```python
from build123d import *

# Parameters (mm, degrees)
BASPROSKE_W         = 2
BASPROSKE_H         = 32
TOOTHCUT_DEPTH      = 46.299006612
TEETHCUTS_COUNT     = 30
TEETHCUTS_ANGLE     = 348
BORSKE_R            = 0.4
BORE_DEPTH          = 50.0000508
CUT_EXTRUDE_1_DEPTH = 10
CUT_EXTRUDE_3_DEPTH = 46.215730311
EXTRUDE_1_DEPTH     = 2
SKETCH_5_R          = 2
CUT_EXTRUDE_4_DEPTH = 10
EXTRUDE_START       = -2
EXTRUDE_2_DEPTH     = 2
SKETCH_8_R          = 2
CUT_EXTRUDE_6_DEPTH = 2
SKETCH_9_R          = 1.5
EXTRUDE_3_DEPTH     = 2
FILLET_7_R          = 2
CUT_EXTRUDE_7_DEPTH = 10
FILLET_8_R          = 2
FILLET_9_R          = 1


with BuildPart() as part:
    # BasProSke → Base-Revolve (revolve)
    with BuildSketch(Plane(origin=(0, 0, 0), x_dir=(1, 0, 0), z_dir=(0, 1, 0)), mode=Mode.PRIVATE) as base_revolve_sk:
        with Locations((1, 16)):
            Rectangle(BASPROSKE_W, BASPROSKE_H)
    revolve(base_revolve_sk.sketch.rotate(Axis((-10, 0, 0), (1, 0, 0)), 180), axis=Axis((-10, 0, 0), (1, 0, 0)))

    # TooCutSke → ToothCut (cut, through all)
    with BuildSketch(Plane(origin=(0, 0, 0), x_dir=(0, 0, -1), z_dir=(1, 0, 0))):
        with BuildLine():
            ThreePointArc((0.918551563, 27.483654488), (0, 27.499), (-0.918551563, 27.483654488))
            ThreePointArc((-0.918551563, 27.483654488), (-1.617208176, 29.787801627), (-2.761784709, 31.906093311))
            ThreePointArc((-2.761784709, 31.906093311), (0, 32.0254), (2.761784709, 31.906093311))
            ThreePointArc((2.761784709, 31.906093311), (1.617208176, 29.787801627), (0.918551563, 27.483654488))
        make_face()
    toothcut = extrude(amount=TOOTHCUT_DEPTH, mode=Mode.SUBTRACT)

    # TeethCuts: ToothCut ×30 about axis
    teethcuts_axis = Axis((-10, 0, 0), (1, 0, 0))
    for i in range(1, TEETHCUTS_COUNT):
        add(toothcut.rotate(teethcuts_axis, i * TEETHCUTS_ANGLE / (TEETHCUTS_COUNT - 1)), mode=Mode.SUBTRACT)

    # BorSke → Bore (cut, symmetric)
    with BuildSketch(Plane(origin=(0, 0, 0), x_dir=(0, 0, -1), z_dir=(1, 0, 0))):
        with Locations(Location((0, 0, 0), (0, 0, 180))):
            Circle(BORSKE_R)
    extrude(amount=BORE_DEPTH, both=True, mode=Mode.SUBTRACT)

    # 草图1 → 切除-拉伸1 (cut)
    with BuildSketch(Plane(origin=(2, 0, 0), x_dir=(0, 0, -1), z_dir=(1, 0, 0))):
        Polygon((3.344910825, 31.824700652), (-3.960111671, -37.677945718), (64.810502564, -34.553326749), (47.008100667, 53.868547869), (5.993727235, 38.229973826), align=None)
    extrude(amount=-CUT_EXTRUDE_1_DEPTH, mode=Mode.SUBTRACT)

    # 草图2 → 切除-拉伸3 (cut, through all)
    with BuildSketch(Plane(origin=(2, 0, 0), x_dir=(0, 0, -1), z_dir=(1, 0, 0))):
        with BuildLine():
            Line((4.939512658, 27.051732213), (6.979218814, 36.725980442))
            Line((6.979218814, 36.725980442), (-6.447162529, 36.725980442))
            Line((-6.447162529, 36.725980442), (-5.501449664, 26.943070586))
            ThreePointArc((-5.501449664, 26.943070586), (-0.286173264, 27.497510903), (4.939512658, 27.051732213))
        make_face()
        with BuildLine():
            Line((-11.106203944, -25.156455135), (-12.164876938, -35.534369935))
            Line((-12.164876938, -35.534369935), (-0.063712698, -31.064954068))
            Line((-0.063712698, -31.064954068), (0, -27.499))
            ThreePointArc((0, -27.499), (-5.675281546, -26.906991292), (-11.106203944, -25.156455135))
        make_face()
    extrude(amount=-CUT_EXTRUDE_3_DEPTH, mode=Mode.SUBTRACT)

    # 草图4 → 凸台-拉伸1 (add)
    with BuildSketch(Plane(origin=(2, 0, 0), x_dir=(0, 0, -1), z_dir=(1, 0, 0))):
        Polygon((2.874428211, 27.348357601), (-2.874428211, -27.348357601), (2.098181265, -27.870999917), (7.847037688, 26.825715284), align=None)
    extrude(amount=-EXTRUDE_1_DEPTH)

    # 草图5 → 切除-拉伸4 (cut)
    with BuildSketch(Plane(origin=(2, 0, 0), x_dir=(0, 0, -1), z_dir=(1, 0, 0))):
        Circle(SKETCH_5_R)
    extrude(amount=-CUT_EXTRUDE_4_DEPTH, mode=Mode.SUBTRACT)

    # 草图6 → 凸台-拉伸2 (add)
    with BuildSketch(Plane(origin=(2, 0, 0), x_dir=(0, 0, -1), z_dir=(1, 0, 0)).offset(EXTRUDE_START)):
        with BuildLine():
            Line((2.874428211, 27.348357601), (7.847037688, 26.825715284))
            ThreePointArc((7.847037688, 26.825715284), (3.170258871, 32.33959835), (-2.125103827, 27.416763754))
            ThreePointArc((-2.125103827, 27.416763754), (0.37622016, 27.496426302), (2.874428211, 27.348357601))
        make_face()
        with BuildLine():
            Line((-2.874428211, -27.348357601), (2.098181265, -27.870999917))
            ThreePointArc((2.098181265, -27.870999917), (-3.622799465, -32.292034417), (-7.778930918, -26.375807756))
            ThreePointArc((-7.778930918, -26.375807756), (-5.348829637, -26.973783986), (-2.874428211, -27.348357601))
        make_face()
    extrude(amount=EXTRUDE_2_DEPTH)

    # 草图8 → 切除-拉伸6 (cut)
    with BuildSketch(Plane(origin=(2, 0, 0), x_dir=(0, 0, -1), z_dir=(1, 0, 0))):
        with Locations((2.87453274, 27.349352123)):
            Circle(SKETCH_8_R)
        with Locations(Location((-2.87453274, -27.349352123, 0), (0, 0, 180))):
            Circle(SKETCH_8_R)
    extrude(amount=-CUT_EXTRUDE_6_DEPTH, mode=Mode.SUBTRACT)

    # 草图9 → 凸台-拉伸3 (add)
    with BuildSketch(Plane(origin=(2, 0, 0), x_dir=(0, 0, -1), z_dir=(1, 0, 0))):
        Polygon((4.375839678, -6.200527675), (20.920655086, 9.776614846), (12.584754641, 18.40869245), (6.327248729, 12.365889233), align=None)
        with Locations((11.248994031, 8.777781877)):
            Circle(SKETCH_9_R, mode=Mode.SUBTRACT)
    extrude(amount=-EXTRUDE_3_DEPTH)

    # 圆角7
    fillet_7_edges = [part.edges().sort_by_distance(p)[0] for p in [
        (1, 27.416763754, 2.125103827),
        (1, -26.375807756, 7.778930918),
        (1, -6.200527675, -4.375839678),
        (1, 18.40869245, -12.584754641),
        (1, 9.776614846, -20.920655086),
    ]]
    fillet(fillet_7_edges, radius=FILLET_7_R)

    # 草图10 → 切除-拉伸7 (cut)
    with BuildSketch(Plane(origin=(2, 0, 0), x_dir=(0, 0, -1), z_dir=(1, 0, 0))):
        with BuildLine():
            Line((0, 22.5), (0, 7.5))
            ThreePointArc((0, 7.5), (-0.978946442, 7.43583646), (-1.941142838, 7.244443697))
            Line((-1.941142838, 7.244443697), (-5.823428515, 21.733331092))
            ThreePointArc((-5.823428515, 21.733331092), (-2.936839325, 22.307509381), (0, 22.5))
        make_face()
        with BuildLine():
            Line((-1.941142838, -7.244443697), (-5.823428515, -21.733331092))
            ThreePointArc((-5.823428515, -21.733331092), (-2.936839325, -22.307509381), (0, -22.5))
            Line((0, -22.5), (0, -7.5))
            ThreePointArc((0, -7.5), (-0.978946442, -7.43583646), (-1.941142838, -7.244443697))
        make_face()
        with BuildLine():
            Line((-4.301823273, -6.143640332), (-12.905469818, -18.430920997))
            ThreePointArc((-12.905469818, -18.430920997), (-15.200779671, -16.588740078), (-17.23599997, -14.462721218))
            Line((-17.23599997, -14.462721218), (-5.745333323, -4.820907073))
            ThreePointArc((-5.745333323, -4.820907073), (-5.066926557, -5.529580026), (-4.301823273, -6.143640332))
        make_face()
        with BuildLine():
            Line((-7.047694656, -2.565151075), (-21.143083968, -7.695453225))
            ThreePointArc((-21.143083968, -7.695453225), (-21.96666016, -4.869891314), (-22.414380707, -1.961004212))
            Line((-22.414380707, -1.961004212), (-7.471460236, -0.653668071))
            ThreePointArc((-7.471460236, -0.653668071), (-7.322220053, -1.623297105), (-7.047694656, -2.565151075))
        make_face()
        with BuildLine():
            Line((-7.471460236, 0.653668071), (-22.414380707, 1.961004212))
            ThreePointArc((-22.414380707, 1.961004212), (-21.96666016, 4.869891314), (-21.143083968, 7.695453225))
            Line((-21.143083968, 7.695453225), (-7.047694656, 2.565151075))
            ThreePointArc((-7.047694656, 2.565151075), (-7.322220053, 1.623297105), (-7.471460236, 0.653668071))
        make_face()
        with BuildLine():
            Line((-5.745333323, 4.820907073), (-17.23599997, 14.462721218))
            ThreePointArc((-17.23599997, 14.462721218), (-15.200779671, 16.588740078), (-12.905469818, 18.430920997))
            Line((-12.905469818, 18.430920997), (-4.301823273, 6.143640332))
            ThreePointArc((-4.301823273, 6.143640332), (-5.066926557, 5.529580026), (-5.745333323, 4.820907073))
        make_face()
    extrude(amount=-CUT_EXTRUDE_7_DEPTH, mode=Mode.SUBTRACT)

    # 圆角8
    # the kernel refuses this fillet: 2 mm, written as the material it adds along each edge
    with BuildSketch(Plane(origin=(2, 21.733331092, 5.823428515), x_dir=(0, -0.9659258262890681, -0.2588190451025213), z_dir=(-1, 0, 0)), Plane(origin=(2, -7.695453225, 21.143083968), x_dir=(0, 0.3420201433256658, -0.9396926207859094), z_dir=(-1, 0, 0)), Plane(origin=(2, -18.430920997, 12.905469818), x_dir=(0, 0.8191520442889906, -0.5735764363510477), z_dir=(-1, 0, 0)), Plane(origin=(2, -22.5, 0), x_dir=(0, 1, 0), z_dir=(-1, 0, 0)), Plane(origin=(2, 14.462721218, 17.23599997), x_dir=(0, -0.6427876096865373, -0.7660444431189798), z_dir=(-1, 0, 0))) as fillet_8_piece_1:
        with BuildLine():
            CenterArc((2.097794237, -2), FILLET_8_R, 90, 95.598737816)
            ThreePointArc((0.107335138, -2.195121951), (0.026849805, -1.098872287), (0, 0))
            Line((0, 0), (2.097794237, 0))
        make_face()
    extrude(amount=2)
    with BuildSketch(Plane(origin=(2, 7.5, 0), x_dir=(0, 1, 0), z_dir=(-1, 0, 0)), Plane(origin=(2, -0.653668071, 7.471460236), x_dir=(0, -0.08715574274765506, 0.9961946980917458), z_dir=(-1, 0, 0)), Plane(origin=(2, -7.244443697, 1.941142838), x_dir=(0, -0.9659258262890681, 0.25881904510252146), z_dir=(-1, 0, 0)), Plane(origin=(2, 2.565151075, 7.047694656), x_dir=(0, 0.3420201433256657, 0.9396926207859094), z_dir=(-1, 0, 0))) as fillet_8_piece_2:
        with BuildLine():
            CenterArc((1.787087811, -2), FILLET_8_R, 90, 77.846802531)
            ThreePointArc((-0.168088571, -1.578947368), (-0.042140531, -0.793934594), (0, 0))
            Line((0, 0), (1.787087811, 0))
        make_face()
    extrude(amount=2)
    with BuildSketch(Plane(origin=(2, 7.244443697, 1.941142838), x_dir=(0, 0.15511388497476047, -0.9878965951394088), z_dir=(-1, 0, 0)), Plane(origin=(2, -2.565151075, 7.047694656), x_dir=(0, 0.9706182844853172, 0.2406244913195247), z_dir=(-1, 0, 0)), Plane(origin=(2, -6.143640332, 4.301823273), x_dir=(0, 0.6570674137305863, 0.7538318206426409), z_dir=(-1, 0, 0)), Plane(origin=(2, -7.5, 0), x_dir=(0, 0.10585794590086138, 0.9943812625395002), z_dir=(-1, 0, 0)), Plane(origin=(2, 4.820907073, 5.745333323), x_dir=(0, 0.6936960644980776, -0.7202678460821911), z_dir=(-1, 0, 0)), Plane(origin=(2, 0.653668071, 7.471460236), x_dir=(0, 0.9813712137228957, -0.1921211619683022), z_dir=(-1, 0, 0))) as fillet_8_piece_3:
        with BuildLine():
            CenterArc((1.79958508, -1.988762525), FILLET_8_R, 96.076598735, 77.846802531)
            Line((-0.189177445, -1.777046633), (0, 0))
            ThreePointArc((0, 0), (0.793934594, -0.042140531), (1.587869189, 0))
        make_face()
    extrude(amount=2)
    with BuildSketch(Plane(origin=(2, -1.961004212, 22.414380707), x_dir=(0, 0.08715574274765493, -0.9961946980917459), z_dir=(-1, 0, 0)), Plane(origin=(2, -21.733331092, 5.823428515), x_dir=(0, 0.9659258262890682, -0.2588190451025213), z_dir=(-1, 0, 0)), Plane(origin=(2, 22.5, 0), x_dir=(0, -1, 0), z_dir=(-1, 0, 0))) as fillet_8_piece_4:
        with BuildLine():
            CenterArc((2.097794237, 2), FILLET_8_R, 174.401262184, 95.598737816)
            ThreePointArc((0.107335138, 2.195121951), (0.026849805, 1.098872287), (0, 0))
            Line((0, 0), (2.097794237, 0))
        make_face()
    extrude(amount=2)
    with BuildSketch(Plane(origin=(2, -14.462721218, 17.23599997), x_dir=(0, -0.7337373482538164, -0.6794332224563776), z_dir=(-1, 0, 0)), Plane(origin=(2, 18.430920997, 12.905469818), x_dir=(0, -0.6128983503496758, 0.7901617632729682), z_dir=(-1, 0, 0)), Plane(origin=(2, 7.695453225, 21.143083968), x_dir=(0, -0.9552751049492566, 0.29571857206504093), z_dir=(-1, 0, 0))) as fillet_8_piece_5:
        with BuildLine():
            CenterArc((2.100067037, -1.997613351), FILLET_8_R, 87.200631092, 95.598737816)
            Line((0.102453687, -2.095290887), (0, 0))
            ThreePointArc((0, 0), (1.098872287, 0.026849805), (2.197744574, 0))
        make_face()
    extrude(amount=2)
    with BuildSketch(Plane(origin=(2, -4.820907073, 5.745333323), x_dir=(0, -0.693696064498077, -0.7202678460821916), z_dir=(-1, 0, 0)), Plane(origin=(2, 6.143640332, 4.301823273), x_dir=(0, -0.6570674137305856, 0.7538318206426414), z_dir=(-1, 0, 0))) as fillet_8_piece_6:
        with BuildLine():
            CenterArc((1.79958508, 1.988762525), FILLET_8_R, 186.076598735, 77.846802531)
            Line((-0.189177445, 1.777046633), (0, 0))
            ThreePointArc((0, 0), (0.793934594, 0.042140531), (1.587869189, 0))
        make_face()
    extrude(amount=2)
    with BuildSketch(Plane(origin=(2, 1.961004212, 22.414380707), x_dir=(0, 0.9907493352683345, -0.1357046597039071), z_dir=(-1, 0, 0))) as fillet_8_piece_7:
        with BuildLine():
            CenterArc((2.100067037, 1.997613351), FILLET_8_R, 177.200631092, 95.598737816)
            Line((0.102453687, 2.095290887), (0, 0))
            ThreePointArc((0, 0), (1.098872287, -0.026849805), (2.197744574, 0))
        make_face()
    extrude(amount=2)

    # 圆角9
    fillet_9_edges = [part.edges().sort_by_distance(p)[0] for p in [
        (1, 12.365889233, -6.327248729),
    ]]
    fillet(fillet_9_edges, radius=FILLET_9_R)


solid = part.part
```
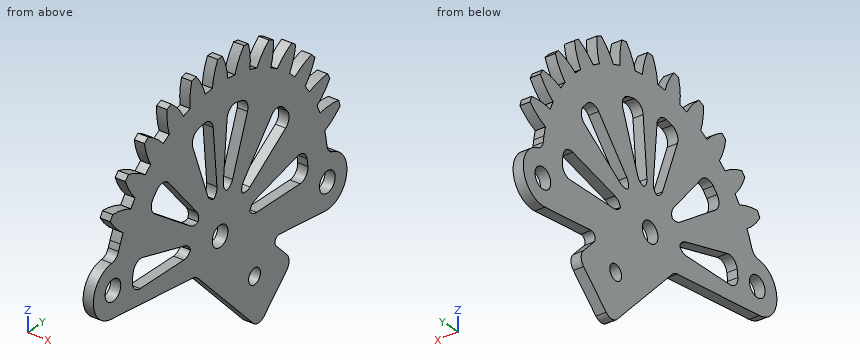
Build history of the part. All positions in model axes, mm. Coordinates: 2 decimals unless noted, no trailing zeros. Order: outer loops, then holes, each group sorted by start corner. A loop starts at its lowest first (then second) coordinate and runs counter-clockwise, first axis right, second up.
Item 1: Drill centre lines: L1, parallel to Z at x = 0.7, y = 27.5; L2, parallel to Z at x = 1.15, y = -27.5; L3, parallel to Z at x = 1.2, y = 22. Where is each one in solid material? Low to high.
Filled in:
L1: z = -7.87 to -4.87, -0.88 to 2.89, 6.99 to 10.62, 14.73 to 16.36
L2: z = -2.14 to 0.88, 4.87 to 7.88, 14.73 to 16.36
L3: z = -7.34 to 0.8, 4.27 to 16.5, 17.24 to 21.42
Item 2: Saw through at B-B on x = 1. State how many separate pieces and enclosed holes the cut face has, then the cut area to 3 significant figures.
Filled in:
separate pieces: 1
enclosed holes: 10
area: 1,510 mm2
Item 3: Drop a flat-ended pin along its axis: pin 1 Ø0.6 at (x, y) = (0.5, 14.5) entering from +Z. Give the stop position or say it passes through.
Filled in:
pin 1: stops at z = 23.63
Item 4: Saw through at A-A on z = 13.5. List the corners of the cut face in (x, y).
Filled in:
outline: (0, -26.47) - (2, -26.47) - (2, -17.56) - (0, -17.56) - close; (0, -11.33) - (2, -11.33) - (2, -4.91) - (0, -4.91) - close; (0, -1.18) - (2, -1.18) - (2, 1.18) - (0, 1.18) - close; (0, 4.91) - (2, 4.91) - (2, 11.33) - (0, 11.33) - close; (0, 17.56) - (2, 17.56) - (2, 26.47) - (0, 26.47) - close
